The model under review builds one solid part; all positions refer to its coordinate system, in mm. Coordinates: 2 decimals unless noted, no trailing zeros. Loops run counter-clockwise (first coordinate to the right, second up) from the corner with the lowest first, then second, coordinate; pieces in that order, holes last. Notation, with made-up numbers: M 44,80 L 93,80 A13 ccw 93,94 Z; hole C 79,15.5 d9. An arc over 180 degrees is marked long. Write item = value, one per line. Start each with the question number.
Q1. Wall thickness on probe 1 along Y at (x, z) = (122, 40); probe 2 along Y at (x, z) = (122.5, 20.5); probe 3 along Y at (x, z) = (115.75, 61.5): over which ranges is each line inside the solid? List them lowest first.
Q2. We need section B-B on z = 46.5. Give the boundary of the cut face in (x, y), and give its area (3 significant figures).
Q3. We need section A-A on x = 122. Give the boundary of the cut face in (y, z).
Q4. Clearance check with flat-ended pins moving along their axes: pin 1 Ø3 at (x, y) = (116, 108.5) entering from +Z; pin 2 Ø1.8 at (x, z) = (117, 34.5) entering from +Y. State where each tip first meets the part, or that it passes through.
Q5. We need section C-C on y = 20. Give the boundary of the cut face in (x, z).
from build123d import *

# Parameters (mm, degrees)
SKETCH025_W             = 75
SKETCH025_H             = 300
PAD008_DEPTH            = 18
SKETCH026_W             = 75
SKETCH026_H             = 18
SKETCH026_W_2           = 57
SKETCH026_H_2           = 12
POCKET017_DEPTH         = 6
SKETCH027_W             = 6
SKETCH027_H             = 6
SKETCH027_W_2           = 3
POCKET018_DEPTH         = 300
SKETCH032_R             = 2.5
POCKET021_DEPTH         = 75
BODY009_PLACEMENT_ANGLE = 90


with BuildPart() as part:
    # Sketch025 → Pad008 (new body)
    with BuildSketch(Plane.XY):
        with Locations((37.5, 150)):
            Rectangle(SKETCH025_W, SKETCH025_H)
    extrude(amount=PAD008_DEPTH)

    # Sketch026 → Pocket017 (cut)
    with BuildSketch(Plane.XY.offset(18)):
        with Locations((37.5, 291)):
            Rectangle(SKETCH026_W, SKETCH026_H)
        with Locations((46.5, 216)):
            Rectangle(SKETCH026_W_2, SKETCH026_H_2)
    extrude(amount=-POCKET017_DEPTH, mode=Mode.SUBTRACT)

    # Sketch027 → Pocket018 (cut)
    with BuildSketch(Plane.XZ):
        with Locations((15, 15)):
            Rectangle(SKETCH027_W, SKETCH027_H)
        with Locations((73.5, 15)):
            Rectangle(SKETCH027_W_2, SKETCH027_H)
    extrude(amount=-POCKET018_DEPTH, mode=Mode.SUBTRACT)

    # Sketch032 → Pocket021 (cut)
    with BuildSketch(Plane.YZ.offset(75)):
        with Locations((20, 9)):
            Circle(SKETCH032_R)
        with Locations((200, 9)):
            Circle(SKETCH032_R)
    extrude(amount=-POCKET021_DEPTH, mode=Mode.SUBTRACT)


with BuildPart() as part_1:
    # Body009 placement: moved
    add(part.part.moved(Location((131, 0, 0))).rotate(Axis((131, 0, 0), (0, -1, 0)), BODY009_PLACEMENT_ANGLE))


solid = part_1.part
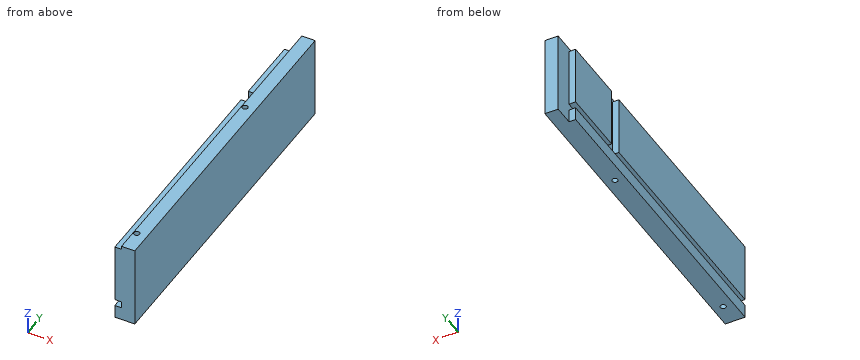
Returned:
q1.probe_1 = 0 to 17.5, 22.5 to 197.5, 202.5 to 300
q1.probe_2 = 0 to 17.55, 22.45 to 197.55, 202.45 to 300
q1.probe_3 = 0 to 210, 222 to 282
q2.outline = M 113,0 L 131,0 L 131,300 L 119,300 L 119,282 L 113,282 L 113,222 L 119,222 L 119,210 L 113,210 Z; hole C 122,20 d5; hole C 122,200 d5
q2.area = 5,180 mm^2
q3.outline = M 0,0 L 17.5,0 L 17.5,75 L 0,75 Z; M 22.5,0 L 197.5,0 L 197.5,75 L 22.5,75 Z; M 202.5,0 L 300,0 L 300,75 L 202.5,75 Z
q4.pin_1 = 72
q4.pin_2 = 282
q5.outline = M 113,0 L 119.5,0 L 119.5,75 L 119,75 L 119,72 L 113,72 L 113,18 L 119,18 L 119,12 L 113,12 Z; M 124.5,0 L 131,0 L 131,75 L 124.5,75 Z
